The model under review builds one solid part; all positions refer to its coordinate system, in mm. Round coordinates to 2 decimals unless told otherwise and drop trailing zeros. Order: outer loops, then holes, each group sorted by start corner. A loop starts at its lowest first (then second) coordinate and runs counter-clockwise, first axis right, second up.
from build123d import *

# Parameters (mm, degrees)
F0_W     = 381
F0_H     = 508
F1_DEPTH = 6.35
F3_D     = 12.7
F3_DEPTH = 25.4


with BuildPart() as f1:
    # F0 (on Top) → F1 (new body)
    with BuildSketch(Plane.XY):
        with Locations((190.5, 254)):
            Rectangle(F0_W, F0_H)
    extrude(amount=F1_DEPTH)

    # F3
    with Locations(Plane.XY.offset(6.35)):
        with Locations((25.4, 12.7), (25.4, 76.2), (292.1, 76.2), (292.1, 12.7)):
            Hole(F3_D / 2, depth=F3_DEPTH)


solid = f1.part
(1) We need section B-B (y = 76.2). Give the boundary of the cut face in (x, z).
(2) To check wall thickness, follow L1, parallel to Y at x = 25.4, z = 3.5. State the ranges of the line that lie inside material, in increasing order.
(3) Clearance check with a flat-ended pin moving along its axis: P1, Ø1.5, axis at x = 178.5, z = 3, coming from the -Y side. State where the tip first meets the part, or that it passes through.
(4) The part is to be moulded in two halves that separate along X. For faces 1 (the cylindrical face through (298.444, 76.479, 3.131)), 2 (the flat face through (188, 258, 6.35)), 3 (the cylindrical face through (21.986, 18.054, 3.131)), say which applies: pulls with the +X half, pulls with the -X half, needs draft (parallel to the pull), parting line crosses it, or undercut.
(5) We need section A-A (x = 25.4). Give the boundary of the cut face in (y, z).
Verdict:
1. outline: (0, 0) - (19.05, 0) - (19.05, 6.35) - (0, 6.35) - close; (31.75, 0) - (285.75, 0) - (285.75, 6.35) - (31.75, 6.35) - close; (298.45, 0) - (381, 0) - (381, 6.35) - (298.45, 6.35) - close
2. L1: y = 0 to 6.35, 19.05 to 69.85, 82.55 to 508
3. P1: stops at y = 0
4. face 1: undercut
4. face 2: needs draft
4. face 3: undercut
5. outline: (0, 0) - (6.35, 0) - (6.35, 6.35) - (0, 6.35) - close; (19.05, 0) - (69.85, 0) - (69.85, 6.35) - (19.05, 6.35) - close; (82.55, 0) - (508, 0) - (508, 6.35) - (82.55, 6.35) - close
